The drawing under review shows one solid part. Ordinate dimensions are in mm from its lowest x, y, z. A direction names the side the tool comes from. Coordinates: 2 decimals unless noted, no trailing zeros. Write each loop counter-clockwise with the first axis right and the second up, starting at its lowest first coordinate (ties: lowest second). Pieces come first, ordered by that corner, then holes.
Q1. For probe 1 along Z at (x, y) = (7.62, 2.5); probe 2 along Z at (x, y) = (23.5, 24.5); probe 3 along Z at (x, y) = (7, 4), list the stretches that pass through material, from the lowest coordinate up.
Q2. Machinability: for the marked faces 1 and 2, which of the approach directions +Z, -Z, +X, -X, +Y, -Y give a long, thin tool a straight path to every point of the face, cutting with its end or side? Answer none if there is none.
Q3. Take a section at A-A (y = 7.62). Give the boundary of the cut face in (x, z) (3 decimals), and give its area (3 significant figures).
Q4. Insertion check: pin 1 (2 mm diameter, centred on x = 4.5, y = 15.5, fed in from +Z); pin 2 (20.5 mm diameter, centred on x = 7.62, z = 7.62, fed in from -Y). Each pin has a flat end and moves straight along its axis. Give the tip position at first contact, or say it passes through.
Q5. Take a section at D-D (x = 16.5). Give the boundary of the cut face in (y, z), and give its area (3 significant figures).
Q6. Take a section at B-B (x = 7.62). Give the boundary of the cut face in (y, z).
Q7. Take a section at C-C (z = 7.62). Give the boundary of the cut face in (x, y), and give its area (3 significant figures).
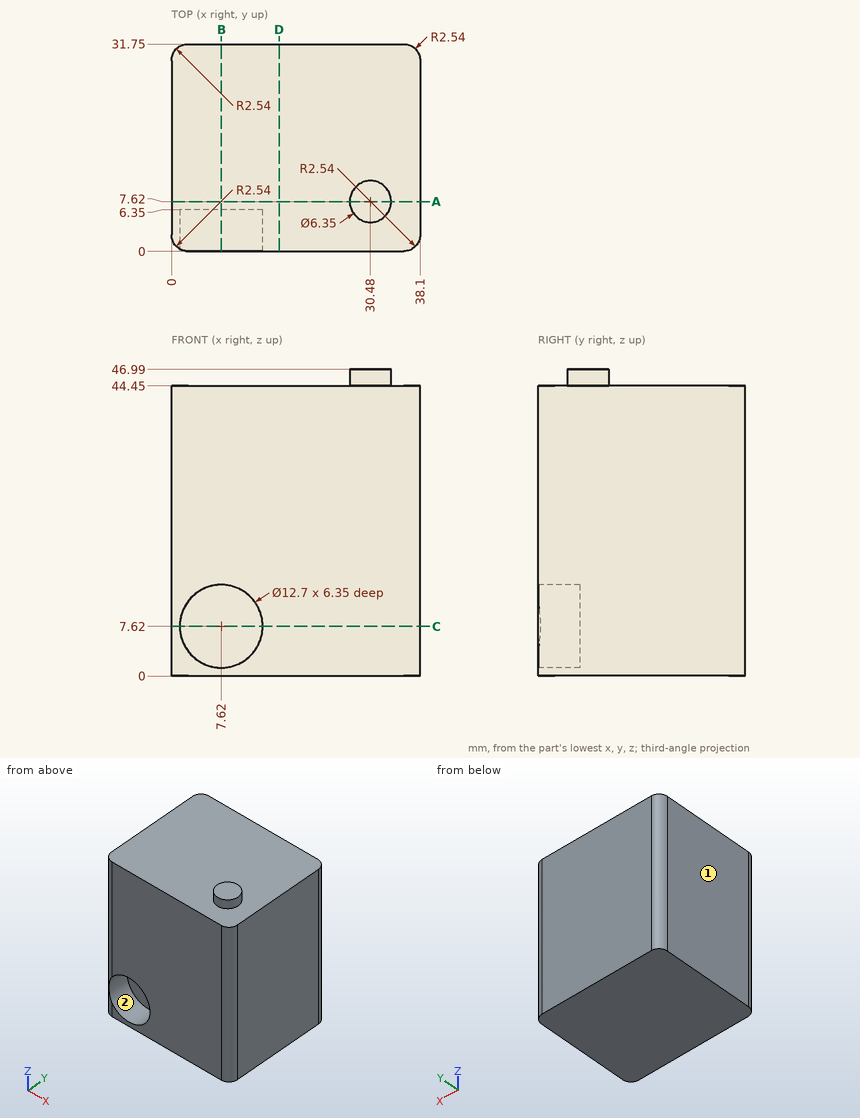
Response:
1. probe 1: z = 0 to 1.27, 13.97 to 44.45
1. probe 2: z = 0 to 44.45
1. probe 3: z = 0 to 1.3, 13.94 to 44.45
2. face 1: +Z, -Z, -X, +Y, -Y
2. face 2: -Y
3. outline: (0, 0) - (38.1, 0) - (38.1, 44.45) - (33.655, 44.45) - (33.655, 46.99) - (27.305, 46.99) - (27.305, 44.45) - (0, 44.45) - close
3. area: 1,710 mm2
4. pin 1: stops at z = 44.45
4. pin 2: stops at y = 0
5. outline: (0, 0) - (31.75, 0) - (31.75, 44.45) - (0, 44.45) - close
5. area: 1,410 mm2
6. outline: (0, 0) - (31.75, 0) - (31.75, 44.45) - (0, 44.45) - (0, 13.97) - (6.35, 13.97) - (6.35, 1.27) - (0, 1.27) - close
7. outline: (0, 2.54) arc R2.54 ccw to (1.27, 0.34) - (1.27, 6.35) - (13.97, 6.35) - (13.97, 0) - (35.56, 0) arc R2.54 ccw to (38.1, 2.54) - (38.1, 29.21) arc R2.54 ccw to (35.56, 31.75) - (2.54, 31.75) arc R2.54 ccw to (0, 29.21) - close
7. area: 1,120 mm2
